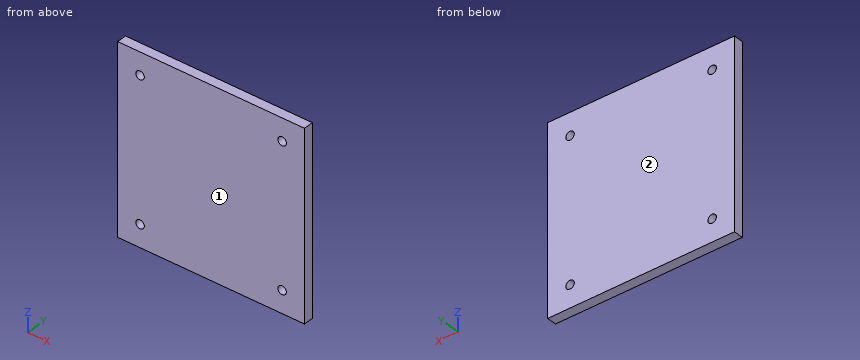
```python
from build123d import *

# Parameters (mm, degrees)
SKETCH1_W                = 38.5
SKETCH1_H                = 38.5
BOSS_EXTRUDE1_DEPTH      = 2
M2_2X0_45_TAPPED_HOLE1_D = 1.75


with BuildPart() as part:
    # Sketch1 → Boss-Extrude1 (new body)
    with BuildSketch(Plane(origin=(0, 0, 0), x_dir=(1, 0, 0), z_dir=(0, 1, 0))):
        with Locations((-0.334475449, -6.202777778)):
            Rectangle(SKETCH1_W, SKETCH1_H)
    extrude(amount=BOSS_EXTRUDE1_DEPTH)

    # M2.2x0.45 Tapped Hole1 (through all)
    with Locations(Plane(origin=(-14.984475449, 2, -8.447222222), x_dir=(0, 0, 1), z_dir=(0, 1, 0))):
        with Locations((0, 0), (29.3, 29.3), (0, 29.3), (29.3, 0)):
            Hole(M2_2X0_45_TAPPED_HOLE1_D / 2)


solid = part.part
```
Part model, mm, in its own coordinate system. Face numbers are marked on the shaded views. Round coordinates to 2 decimals unless told otherwise and drop trailing zeros.
1. Two-plate mould, pull along Y, no slides. Class the marked faces 1 and 2: pulls with the +Y half, pulls with the -Y half, needs draft (parallel to the pull), parting line crosses it, or undercut.
Solutions:
face 1: pulls with the -Y half
face 2: pulls with the +Y half
2. Flat gauge pin, fed straight in: pin 1 (1.6 mm diameter, centred on x = 14.32, z = 20.85, fed in from +Y). Where does the tip first touch, or does it go through?
Solutions:
pin 1: passes through
3. Drill centre lines: line 1 along X through (y, z) = (0.45, 21); line 2 along Z through (x, y) = (-15.5, 1.7); line 3 along X through (y, z) = (1.85, 21.5). Where is each one in solid material? Low to high.
Solutions:
line 1: x = -19.58 to -15.85, -14.12 to 13.45, 15.18 to 18.92
line 2: z = -13.05 to -9.15, -7.74 to 20.15, 21.56 to 25.45
line 3: x = -19.58 to -15.57, -14.4 to 13.73, 14.9 to 18.92
